Autodesk Inventor part; units mm, degrees
ref_plane "YZ Plane" through (0, 0, 0) normal (1, 0, 0) x (0, 1, 0)
ref_plane "XZ Plane" through (0, 0, 0) normal (0, 1, 0) x (-1, 0, 0)
ref_plane "XY Plane" through (0, 0, 0) normal (0, 0, 1) x (1, 0, 0)
sketch "Sketch1" plane through (0, 0, 0) normal (1, 0, 0) x (0, 1, 0)
  line L0 (4.475, 0.31) -> (-4.475, 0.31)
  line L1 (-4.475, 0.31) -> (-4.475, -0.31)
  line L2 (-4.475, -0.31) -> (4.475, -0.31)
  line L3 (4.475, -0.31) -> (4.475, 0.31)
  line L4 (4.475, 0.31) -> (-4.475, -0.31) construction
  line L5 (-4.475, 0.31) -> (4.475, -0.31) construction
  point P0 (0, 0)
  dimension "d0" = 8.95
  dimension "d1" = 0.62
extrude "Extrusion1" add sketch "Sketch1" along normal blind 0.62
chamfer "Chamfer1" distance 0.35 angle 25 1 edges at (0.31, 4.475, 0.31) measured on face at (0.4133, 1.4917, 0.31)
chamfer "Chamfer2" distance 0.35 angle 25 1 edges at (0.62, 4.475, -0.0816) measured on face at (0.62, 1.375, -0.1033)
chamfer "Chamfer3" distance 0.35 angle 25 1 edges at (0.2284, 4.475, -0.31) measured on face at (0.2067, 1.375, -0.31)
chamfer "Chamfer4" distance 0.35 angle 25 1 edges at (0, 4.475, 0) measured on face at (0, 1.2583, -0.1033)
chamfer "Chamfer5" distance 0.35 angle 25 1 edges at (0.31, -4.475, -0.31) measured on face at (0.2067, -1.6083, -0.31)
chamfer "Chamfer6" distance 0.35 angle 25 1 edges at (0.62, -4.475, 0.0816) measured on face at (0.62, -1.4917, 0.1033)
chamfer "Chamfer7" distance 0.35 angle 25 1 edges at (0.2284, -4.475, 0.31) measured on face at (0.2067, -1.4917, 0.31)
chamfer "Chamfer8" distance 0.35 angle 25 1 edges at (0, -4.475, 0) measured on face at (0, 1.375, -0.1033)
properties part number "Pin_Header" material "Nickel-Copper Alloy 400"
Input: part model. Units: mm. Frame: model coordinates. Coordinates: 2 decimals unless noted, no trailing zeros. Loops run counter-clockwise (first coordinate to the right, second up) from the corner with the lowest first, then second, coordinate; pieces in that order, holes last.
Q1. Section B-B, the plane z = 0.05. Return the cut outline in (x, y) (3 decimals).
Results are:
outline: (0, -4.125) - (0.163, -4.475) - (0.457, -4.475) - (0.62, -4.125) - (0.62, 4.125) - (0.457, 4.475) - (0.163, 4.475) - (0, 4.125) - close
Q2. Line query: line 1 along Z through (x, y) = (0.15, 4.25); line 2 along Y through (x, z) = (0.2, -0.2); line 3 along Y through (x, z) = (0.3, -0.25). Output: solid intervals per line, ascending.
Results are:
line 1: z = -0.25 to 0.25
line 2: y = -4.36 to 4.36
line 3: y = -4.25 to 4.25
Q3. Section A-A, the plane x = 0.3. Return the cut outline in (y, z) (3 decimals).
Results are:
outline: (-4.475, -0.147) - (-4.125, -0.31) - (4.125, -0.31) - (4.475, -0.147) - (4.475, 0.147) - (4.125, 0.31) - (-4.125, 0.31) - (-4.475, 0.147) - close
